CAD build for the part. Positions are in the model's coordinates, mm. Coordinates: 2 decimals unless noted, no trailing zeros. Write each loop counter-clockwise with the first axis right and the second up, starting at its lowest first coordinate (ties: lowest second). Pieces come first, ordered by that corner, then holes. Notation, with made-up numbers: (83, 53.5) - (124, 53.5) arc R11 cw to (124, 58.5) - close; hole circle Ø6 at (31.5, 28.5). An arc over 180 degrees is marked (long way). One line per question, with ' | ' between items. Start each with the question number.
1. Probe line 1 (Y direction, x = 0, z = 5.5); line 2 (Y direction, x = 2, z = 4.75); line 3 (Z direction, x = 1.5, y = -2). List the from-to ranges inside material, lowest first.
2. Band-saw the part on C-C, the plane z = 3.25. Write the cut outline in (x, y), then the cut area to 3 significant figures.
3. Flat gauge pins, fed straight in: P1, Ø1, axis at x = -2.5, y = -0.5, coming from the -Z side; P2, Ø3, axis at x = -1, y = -1, coming from the -Z side; P3, Ø2, axis at y = -5, z = 8, coming from the -X side; P4, Ø2, axis at x = 2.5, z = 4, coming from the +Y side. Where does each tip first touch, or does it go through?
4. Band-saw the part on A-A, the plane x = 0. Write the cut outline in (y, z).
5. Band-saw the part on D-D, the plane z = 16. Write the cut outline in (x, y).
6. Two-plate mould, pull along X, no slides. Class faces 1 (the flat face through (0, 0, 20)), 2 (the cylindrical face through (-3, 0, 5)), 3 (the cylindrical face through (-7.493, 0.33, 8.874)), 4 (the flat face through (0, 0, 10)): +X half, -X half, draft (parallel to the pull), parting line (faces both ways), or undercut.
from build123d import *

# Parameters (mm, degrees)
F0_R     = 7.5
F1_DEPTH = 20
F2_SIZE  = 2
F3_R     = 3
F4_DEPTH = 10


with BuildPart() as f1:
    # F0 (on Top) → F1 (new body)
    with BuildSketch(Plane.XY):
        Circle(F0_R)
    extrude(amount=F1_DEPTH)

    # F2
    f2_edges = [f1.edges().sort_by_distance(p)[0] for p in [
        (-7.5, 0, 20),
    ]]
    chamfer(f2_edges, length=F2_SIZE)

    # F3 (on face) → F4 (cut)
    with BuildSketch(Plane(origin=(0, 0, 0), x_dir=(1, 0, 0), z_dir=(0, 0, -1))):
        Circle(F3_R)
    extrude(amount=-F4_DEPTH, mode=Mode.SUBTRACT)


solid = f1.part
Filled in:
1) line 1: y = -7.5 to -3, 3 to 7.5 | line 2: y = -7.23 to -2.24, 2.24 to 7.23 | line 3: z = 10 to 20
2) outline: circle Ø15 at (0, 0); hole circle Ø6 at (0, 0) | area: 148 mm²
3) P1: stops at z = 0 | P2: stops at z = 10 | P3: stops at x = -6.34 | P4: stops at y = 7.35
4) outline: (-7.5, 0) - (-3, 0) - (-3, 10) - (3, 10) - (3, 0) - (7.5, 0) - (7.5, 18) - (5.5, 20) - (-5.5, 20) - (-7.5, 18) - close
5) outline: circle Ø15 at (0, 0)
6) face 1: draft | face 2: undercut | face 3: parting line | face 4: undercut
